```python
from build123d import *

# Parameters (mm, degrees)
F0_W     = 81
F0_H     = 9
F1_DEPTH = 25
F2_W     = 81
F2_H     = 0.2
F3_DEPTH = 7.85
F4_W     = 40.5
F4_H     = 2.5
F5_DEPTH = 85
F7_DEPTH = 25


with BuildPart() as f1:
    # F0 (on Top) → F1 (new body)
    with BuildSketch(Plane.XY):
        with Locations((40.5, 4.5)):
            Rectangle(F0_W, F0_H)
    extrude(amount=F1_DEPTH)

    # F2 (on face) → F3 (cut)
    with BuildSketch(Plane(origin=(0, 0, 0), x_dir=(1, 0, 0), z_dir=(0, 0, -1))):
        with Locations((40.5, -4.5)):
            Rectangle(F2_W, F2_H)
    extrude(amount=-F3_DEPTH, mode=Mode.SUBTRACT)

    # F4 (on face) → F5 (join)
    with BuildSketch(Plane.XY.offset(25)):
        with Locations((20.25, 5.75)):
            Rectangle(F4_W, F4_H)
        with Locations((20.25, 3.25)):
            Rectangle(F4_W, F4_H)
        with Locations((60.75, 3.25)):
            Rectangle(F4_W, F4_H)
        with Locations((60.75, 5.75)):
            Rectangle(F4_W, F4_H)
    extrude(amount=F5_DEPTH)

    # F6 (on face) → F7 (cut)
    with BuildSketch(Plane.XZ.offset(-2)):
        Polygon((0, 110), (0, 40), (20.25, 47.5), (20.25, 110), align=None)
        Polygon((60.75, 47.5), (81, 40), (81, 110), (60.75, 110), align=None)
    extrude(amount=-F7_DEPTH, mode=Mode.SUBTRACT)


solid = f1.part
```
Geometry: final body of the model. Coordinates: model frame, mm. A direction names the side the tool comes from. Coordinates: 2 decimals unless noted, no trailing zeros. Write each loop counter-clockwise with the first axis right and the second up, starting at its lowest first coordinate (ties: lowest second). Pieces come first, ordered by that corner, then holes. Notation, with made-up numbers: M 55,-8 L 85,-8 A11 cw 85,-4 Z; hole C 30,43 d4. An arc over 180 degrees is marked long. Use CSV: the item, a comma, the result in double quotes. Start each with the question number.
1. Reachability of faces 1 (the face through (20.25, 4, 78)), 2 (the face through (40, 2, 57)), 3 (the face through (40, 4.6, 4)) from +Z, -Z, +X, -X, +Y, -Y: full face, straight path, thin tool, end or side. Return the list, or none.
2. Cut plane A-A on x = 57. Return the cut outline in (y, z).
3. Mould query, pull axis Y, two halves, no side actions, for faces 4 (the face through (40, 9, 12)), 5 (the face through (40, 7, 0)), 6 (the face through (40, 4.4, 4)). Classes: pulls with the +Y half, pulls with the -Y half, needs draft (parallel to the pull), parting line crosses it, or undercut.
4. Cut plane C-C on x = 69. Return the cut outline in (y, z), plus the area to 3 significant figures.
5. First-contact query: P1, Ø0.6, axis at x = 39.5, y = 0.5, coming from the +Z side; P2, Ø1, axis at y = 6, z = 54, coming from the -X side; P3, Ø4, axis at x = 15.5, y = 7, coming from the +Z side. Flat tips, straight axial feed; report the tip coordinate or a pass-through.
6. Ray query, probe 1 along X at (y, z) = (3.25, 51); probe 2 along Y at (x, z) = (43.5, 40.5); probe 3 along Z at (x, y) = (7, 8.5). Return the intervals inside material, ascending.
7. Cut plane D-D on z = 54.5. Return the cut outline in (x, y).
8. Cut plane B-B on z = 37. Return the cut outline in (x, y).
Entries:
1,face 1,"+Z, -X, +Y, -Y"
1,face 2,"+Z, +X, -X, -Y"
1,face 3,"-Z, +X, -X"
2,outline,"M 0,0 L 4.4,0 L 4.4,7.85 L 4.6,7.85 L 4.6,0 L 9,0 L 9,25 L 7,25 L 7,110 L 2,110 L 2,25 L 0,25 Z"
3,face 4,"pulls with the +Y half"
3,face 5,"needs draft"
3,face 6,"undercut"
4,outline,"M 0,0 L 4.4,0 L 4.4,7.85 L 4.6,7.85 L 4.6,0 L 9,0 L 9,25 L 7,25 L 7,44.44 L 2,44.44 L 2,25 L 0,25 Z"
4,area,"321 mm²"
5,P1,"z = 25"
5,P2,"x = 20.25"
5,P3,"z = 46.48"
6,probe 1,"20.25 to 60.75"
6,probe 2,"2 to 7"
6,probe 3,"0 to 25"
7,outline,"M 20.25,2 L 60.75,2 L 60.75,7 L 20.25,7 Z"
8,outline,"M 0,2 L 81,2 L 81,7 L 0,7 Z"
